Read the model definition and answer for the solid it produces. Units are mm, in the model's axes. A direction names the side the tool comes from. Coordinates: 2 decimals unless noted, no trailing zeros. Order: outer loops, then holes, each group sorted by start corner. A loop starts at its lowest first (then second) coordinate and runs counter-clockwise, first axis right, second up. Notation, with made-up numbers: M -38,59.5 L 15,59.5 A22 cw 15,83.5 Z; hole C -11,84 d10. An arc over 180 degrees is marked long. One line per question, with ' | ' between items. Start each with the question number.
1) Find section B-B, the plane x = 9. Write down the section's boundary in (y, z).
2) Given P1, Ø3, axis at y = -7, z = 10, coming from the -X side; P2, Ø6, axis at y = -149, z = 1.5, coming from the +X side; P3, Ø3, axis at y = -106, z = 5.5, coming from the -X side, each flat-ended and moving along its own axis, determine where each tip first touches the part or whether it passes through.
3) A tool of negligible diameter and unlimited length cuts with its end or side. For faces 1 (the face through (-6.99, -77.87, 7.4)), 2 (the face through (-14, -36, 7)), 3 (the face through (20.252, -53.596, 7.395)), 4 (the face through (19, -96, 15)), from which of +Z, -Z, +X, -X, +Y, -Y can it reach the whole face along a straight path? Write none if from no direction.
4) Consider probe 1 along Y at (x, z) = (-9.5, 2.25); probe 2 along Y at (x, z) = (21, 4.25); probe 3 along Y at (x, z) = (-16.5, 3.25). Determine where each line is inside the solid, lowest interval first.
5) Find section A-A, the plane y = 0. Write down the section's boundary in (x, z).
6) The mould has two halves that part along Y. Classify faces 5 (the face through (19, -96, 0)), 6 (the face through (11.923, 3.755, 7.395)), 7 (the face through (-54.52, -87.33, 7.4)), 8 (the face through (13.15, -141.26, 7.4)): +Y half, -Y half, draft (parallel to the pull), parting line (faces both ways), or undercut.
7) Find section D-D, the plane y = -131.5. Write down the section's boundary in (x, z), plus the area to 3 significant figures.
8) Find section C-C, the plane z = 6.25. Write down the section's boundary in (x, y), plus the area to 3 significant figures.
from build123d import *

# Parameters (mm, degrees)
SKETCH_R  = 12.5
PAD_DEPTH = 15


with BuildPart() as part:
    # Sketch → Pad (new body)
    with BuildSketch(Plane.XY):
        with BuildLine():
            ThreePointArc((-24.759708, -123.457867), (13.746972, -140.88111), (12.962963, -98.62334))
            ThreePointArc((-14, -50.739622), (-6.795871, -78.216211), (12.962963, -98.62334))
            Line((-14, -22.248595), (-14, -50.739622))
            ThreePointArc((-14, -22.248595), (-14.310736, -20.918988), (-15.178571, -19.864817))
            ThreePointArc((15.178571, -19.864817), (0, 25), (-15.178571, -19.864817))
            ThreePointArc((15.178571, -19.864817), (14.310736, -20.918988), (14, -22.248595))
            Line((14, -22.248595), (14, -29.385432))
            ThreePointArc((14, -29.385432), (20.427246, -53.909198), (38.056604, -72.128153))
            ThreePointArc((-46.999155, -119.692368), (36.33247, -168.876744), (38.056604, -72.128153))
            ThreePointArc((-46.999155, -119.692368), (-49.050241, -107.16628), (-55.112152, -96.014461))
            ThreePointArc((-46.031526, -86.852067), (-54.616749, -87.424453), (-55.112152, -96.014461))
            ThreePointArc((-24.759708, -123.457867), (-31.802947, -103.067248), (-46.031526, -86.852067))
        make_face()
        Circle(SKETCH_R, mode=Mode.SUBTRACT)
    extrude(amount=PAD_DEPTH)


solid = part.part
Report:
1) outline: M -176,0 L -143.32,0 L -143.32,15 L -176,15 Z; M -95.98,0 L -8.67,0 L -8.67,15 L -95.98,15 Z; M 8.67,0 L 23.32,0 L 23.32,15 L 8.67,15 Z
2) P1: stops at x = -24.39 | P2: stops at x = 58.6 | P3: stops at x = -50.08
3) face 1: +Z, -Z | face 2: +Z, -Z, -X | face 3: +Z, -Z, +X | face 4: +Z, +X, -X, +Y, -Y
4) probe 1: y = -172.86 to -143.12, -72.73 to -8.12, 8.12 to 23.12 | probe 2: y = -174.7 to -133.56, -106.44 to -54.9, -13.56 to 13.56 | probe 3: y = -169.86 to -138.78, -18.78 to 18.78
5) outline: M -25,0 L -12.5,0 L -12.5,15 L -25,15 Z; M 12.5,0 L 25,0 L 25,15 L 12.5,15 Z
6) face 5: draft | face 6: undercut | face 7: parting line | face 8: undercut
7) outline: M -45.81,0 L -22.2,0 L -22.2,15 L -45.81,15 Z; M 22.2,0 L 63.81,0 L 63.81,15 L 22.2,15 Z | area: 978 mm^2
8) outline: M -55.11,-96.01 A38 cw -47,-119.69 A56 ccw long 38.06,-72.13 A50 cw 14,-29.39 L 14,-22.25 A3 cw 15.18,-19.86 A25 ccw long -15.18,-19.86 A3 cw -14,-22.25 L -14,-50.74 A56 ccw 12.96,-98.62 A25 cw long -24.76,-123.46 A56 ccw -46.03,-86.85 A6.5 ccw Z; hole C 0,0 d25 | area: 9,960 mm^2
